Part model, mm, in its own coordinate system. Coordinates: 2 decimals unless noted, no trailing zeros. Write item = value, one per line. Start each with the question number.
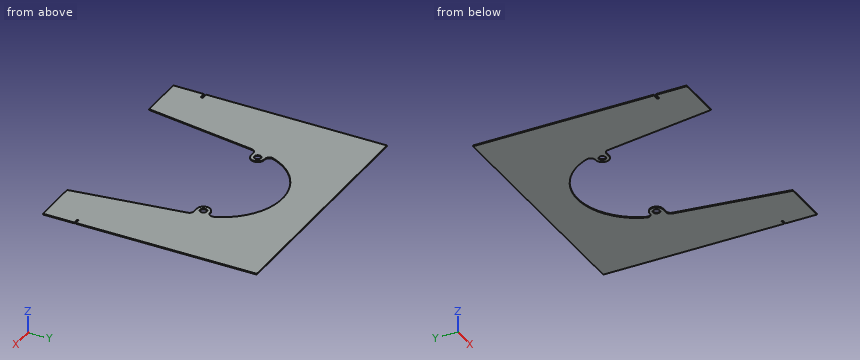
from build123d import *

# Parameters (mm, degrees)
SKETCH1_R           = 9.592533987
SKETCH1_R_2         = 9.525
BOSS_EXTRUDE1_DEPTH = 2.54


with BuildPart() as part:
    # Sketch1 → Boss-Extrude1 (new body)
    with BuildSketch(Plane.XY):
        with BuildLine():
            Line((325.101849056, -276.74558404), (325.101849056, -188.761052666))
            Line((325.101849056, -188.761052666), (311.147367129, -188.761052666))
            Line((311.147367129, -188.761052666), (311.147367129, -184.170327252))
            Line((311.147367129, -184.170327252), (325.101849056, -184.170327252))
            Line((325.101849056, -184.170327252), (325.101849056, 325.138013642))
            Line((325.101849056, 325.138013642), (-361.55061518, 325.138013642))
            Line((-361.55061518, 325.138013642), (-361.55061518, -184.170327252))
            Line((-361.55061518, -184.170327252), (-344.367661442, -184.170327252))
            Line((-344.367661442, -184.170327252), (-344.367661442, -190.835742865))
            Line((-344.367661442, -190.835742865), (-361.55061518, -190.835742865))
            Line((-361.55061518, -190.835742865), (-361.55061518, -276.74558404))
            Line((-361.55061518, -276.74558404), (-234.55061518, -276.74558404))
            add(Edge.make_bspline(
                [(-187.980509507, 38.133773771), (-188.27489671, 36.13210674), (-188.569257118, 34.130435751), (-190.3693668, 21.889980342), (-191.876305024, 11.651371561), (-196.404427488, -19.063375229), (-199.428229196, -39.539126569), (-205.483427481, -80.489507286), (-208.515826842, -100.963988527), (-219.215042163, -173.207603441), (-226.881928481, -224.976726722), (-234.55061518, -276.74558404)],
                knots=[0.775140665, 0.775140665, 0.775140665, 0.775140665, 0.78125, 0.78125, 0.8125, 0.8125, 0.875, 0.875, 0.9375, 0.9375, 1.095529214, 1.095529214, 1.095529214, 1.095529214], degree=3))
            ThreePointArc((-187.980509507, 38.133773771), (-183.716916528, 45.897266013), (-175.41567054, 48.985850142))
            Line((-175.41567054, 48.985850142), (-161.253773138, 48.985850142))
            ThreePointArc((-161.253773138, 48.985850142), (-142.203773138, 68.035850142), (-161.253773138, 87.085850141))
            Line((-161.253773138, 87.085850141), (-162.853778681, 87.085850141))
            ThreePointArc((-162.853778681, 87.085850141), (-173.256071513, 92.500089794), (-174.788993269, 104.126432214))
            add(Edge.make_bspline(
                [(138.340023196, 104.1264177), (138.155537808, 104.633695525), (137.968537838, 105.140328765), (136.878523505, 108.050508672), (135.441958767, 111.634797813), (133.873557403, 115.185292105), (132.798253571, 117.544674285), (132.244938124, 118.72221102), (129.414540718, 124.567063869), (126.94937257, 129.101743153), (121.630471343, 137.897930344), (118.776746577, 142.159444094), (112.686474548, 150.413337301), (107.831924529, 156.402096918), (102.540177193, 162.083495309), (99.819602382, 164.871677634), (98.900271279, 165.792240869), (97.046227751, 167.606080988), (96.110329243, 168.500592287), (91.386634358, 172.911358508), (87.466457166, 176.242558862), (79.351868776, 182.521609038), (75.1575089, 185.469530602), (66.495709426, 190.983636766), (62.02828952, 193.549848892), (55.115179884, 197.102841468), (52.770906129, 198.23944579), (48.057920232, 200.390162802), (45.684402026, 201.406997485), (38.513619271, 204.284843788), (33.666257106, 205.973646323), (23.839984133, 208.89905679), (18.861006507, 210.13543504), (11.293001851, 211.647842714), (8.753729317, 212.094901761), (4.919604431, 212.678810774), (3.63735506, 212.858983123), (1.064351829, 213.190093886), (-0.227403309, 213.341124006), (-4.104657388, 213.748796074), (-6.69392087, 213.960280793), (-10.584377098, 214.188154302), (-11.882288513, 214.24923116), (-14.480247284, 214.34229574), (-15.77998427, 214.375695042), (-18.379751713, 214.405675513), (-19.679864546, 214.392033292), (-22.279014783, 214.333304532), (-23.578445595, 214.289247872), (-27.473045877, 214.113425657), (-30.064936685, 213.93719921), (-35.239513244, 213.464285113), (-37.82599866, 213.167115032), (-42.960254521, 212.456338993), (-45.510284017, 212.042773536), (-53.109929228, 210.630443886), (-58.109124925, 209.46012554), (-67.974579463, 206.667171099), (-72.840887694, 205.044703051), (-80.039629101, 202.268297913), (-83.613765485, 200.794235552), (-87.149475357, 199.189426954), (-89.497993793, 198.090219969), (-90.669429689, 197.525202002), (-96.484812077, 194.636054099), (-100.994154698, 192.125739674), (-109.738071064, 186.722649456), (-113.972669304, 183.829907758), (-122.167753951, 177.662877555), (-126.128054678, 174.388330596), (-131.857503737, 169.182808313), (-133.731998876, 167.398469262), (-136.490242047, 164.64749262), (-137.400625577, 163.718129876), (-139.194142166, 161.84440698), (-140.078494423, 160.898848159), (-144.439064905, 156.128155654), (-147.732037091, 152.174555571), (-153.934907403, 143.998797648), (-156.844744983, 139.776597363), (-162.276947412, 131.060555304), (-164.799263726, 126.566679506), (-168.283130528, 119.615822968), (-169.395978502, 117.259661658), (-171.499158951, 112.524180704), (-172.492247577, 110.139827958), (-173.895945336, 106.538995231), (-174.349562031, 105.334727793), (-174.788993269, 104.126432214)],
                knots=[0.295230777, 0.295230777, 0.295230777, 0.295230777, 0.296875, 0.296875, 0.3046875, 0.30859375, 0.30859375, 0.3125, 0.3125, 0.328125, 0.328125, 0.34375, 0.34375, 0.359375, 0.3671875, 0.3671875, 0.37109375, 0.37109375, 0.375, 0.375, 0.390625, 0.390625, 0.40625, 0.40625, 0.421875, 0.421875, 0.4296875, 0.4296875, 0.4375, 0.4375, 0.453125, 0.453125, 0.46875, 0.46875, 0.4765625, 0.4765625, 0.48046875, 0.48046875, 0.484375, 0.484375, 0.4921875, 0.4921875, 0.49609375, 0.49609375, 0.5, 0.5, 0.50390625, 0.50390625, 0.5078125, 0.5078125, 0.515625, 0.515625, 0.5234375, 0.5234375, 0.53125, 0.53125, 0.546875, 0.546875, 0.5625, 0.5625, 0.5703125, 0.57421875, 0.57421875, 0.578125, 0.578125, 0.59375, 0.59375, 0.609375, 0.609375, 0.625, 0.625, 0.6328125, 0.6328125, 0.63671875, 0.63671875, 0.640625, 0.640625, 0.65625, 0.65625, 0.671875, 0.671875, 0.6875, 0.6875, 0.6953125, 0.6953125, 0.703125, 0.703125, 0.707030961, 0.707030961, 0.707030961, 0.707030961], degree=3))
            ThreePointArc((138.340023196, 104.1264177), (136.807091731, 92.500083469), (126.404803329, 87.085850141))
            Line((126.404803329, 87.085850141), (124.418789558, 87.085850141))
            ThreePointArc((124.418789558, 87.085850141), (105.368789558, 68.035850142), (124.418789558, 48.985850142))
            Line((124.418789558, 48.985850142), (138.966782744, 48.985850142))
            ThreePointArc((138.966782744, 48.985850142), (147.268029336, 45.897265491), (151.531621943, 38.133772192))
            add(Edge.make_bspline(
                [(198.101849056, -276.74558404), (190.457207742, -225.140201219), (182.814584349, -173.534519662), (172.163765006, -101.617813639), (169.155561459, -81.306790297), (163.148374331, -40.683378675), (160.148663276, -20.371098521), (155.656220674, 10.098370509), (154.16095032, 20.255186016), (152.288653907, 32.986071489), (151.910159921, 35.559925083), (151.531621943, 38.133772192)],
                knots=[-0.096298018, -0.096298018, -0.096298018, -0.096298018, 0.0625, 0.0625, 0.125, 0.125, 0.1875, 0.1875, 0.21875, 0.21875, 0.22666892, 0.22666892, 0.22666892, 0.22666892], degree=3))
            Line((198.101849056, -276.74558404), (325.101849056, -276.74558404))
        make_face()
        with Locations((-161.253773138, 68.035850142)):
            Circle(SKETCH1_R, mode=Mode.SUBTRACT)
        with Locations((124.418789558, 68.035850142)):
            Circle(SKETCH1_R_2, mode=Mode.SUBTRACT)
    extrude(amount=BOSS_EXTRUDE1_DEPTH)


solid = part.part
Item 1: Cut at A-A, the plane z = 1.7. Count the separate pieces of the cut face and the enclosed holes in it, and give its area (3 significant figures).
Item 2: Flat gauge pins, fed straight in: pin 1 (17 mm diameter, centred on x = 124.42, y = 68.04, fed in from -Z); pin 2 (0.8 mm diameter, centred on y = -186, z = 1, fed in from -X); pin 3 (0.8 mm diameter, centred on x = 133.5, z = 1.5, fed in from -Y). Where does each tip first touch, or does it go through?
Item 3: Wall check: line 1 along X through (y, z) = (-149.5, 2.3); line 2 along X through (y, z) = (-136, 1.45); line 3 along Y through (x, z) = (-151, 2.2). Give the ranges that are in metal, low to high. Write a range as [from, to].
Filled sheet:
q1.separate_pieces = 1
q1.enclosed_holes = 2
q1.area = 247,000 mm2
q2.pin_1 = through
q2.pin_2 = -344.37
q2.pin_3 = 48.99
q3.line_1 = [-361.55, -215.7], [179.26, 325.1]
q3.line_2 = [-361.55, -213.7], [177.26, 325.1]
q3.line_3 = [51.98, 84.09], [147.87, 325.14]
